from build123d import *

# Parameters (mm, degrees)
SKETCH1_W           = 5
SKETCH1_H           = 30
SKETCH1_W_2         = 30
SKETCH1_H_2         = 5.002209569
BOSS_EXTRUDE2_DEPTH = 5
FILLET1_R           = 5
FILLET2_R           = 2.5


with BuildPart() as part:
    # Sketch1 → Boss-Extrude2 (new body)
    with BuildSketch(Plane.XY):
        with BuildLine():
            Line((-77.831835846, -13.494171848), (-37.831835846, -13.494171848))
            ThreePointArc((-37.831835846, -13.494171848), (-30.760768034, -10.56523966), (-27.831835846, -3.494171848))
            Line((-27.831835846, -3.494171848), (-15.331835846, -3.494171848))
            Line((-15.331835846, -3.494171848), (-15.331835846, 36.505828152))
            Line((-15.331835846, 36.505828152), (-27.831835846, 36.505828152))
            ThreePointArc((-27.831835846, 36.505828152), (-30.760768034, 43.576895964), (-37.831835846, 46.505828152))
            Line((-37.831835846, 46.505828152), (-37.831835846, 59.005828152))
            Line((-37.831835846, 59.005828152), (-77.831835846, 59.005828152))
            Line((-77.831835846, 59.005828152), (-77.831835846, 46.505828152))
            ThreePointArc((-77.831835846, 46.505828152), (-84.902903658, 43.576895964), (-87.831835846, 36.505828152))
            Line((-87.831835846, 36.505828152), (-100.331835846, 36.505828152))
            Line((-100.331835846, 36.505828152), (-100.331835846, -3.494171848))
            Line((-100.331835846, -3.494171848), (-87.831835846, -3.494171848))
            ThreePointArc((-87.831835846, -3.494171848), (-84.902903658, -10.56523966), (-77.831835846, -13.494171848))
        make_face()
        with Locations((-90.331835846, 16.505828152)):
            Rectangle(SKETCH1_W, SKETCH1_H, mode=Mode.SUBTRACT)
        with Locations((-57.831835846, 49.006932937)):
            Rectangle(SKETCH1_W_2, SKETCH1_H_2, mode=Mode.SUBTRACT)
        with Locations((-25.331835846, 16.505828152)):
            Rectangle(SKETCH1_W, SKETCH1_H, mode=Mode.SUBTRACT)
    extrude(amount=BOSS_EXTRUDE2_DEPTH)

    # Fillet1
    fillet1_edges = [part.edges().sort_by_distance(p)[0] for p in [
        (-15.331835846, 36.505828152, 2.5),
        (-15.331835846, -3.494171848, 2.5),
        (-100.331835846, -3.494171848, 2.5),
        (-100.331835846, 36.505828152, 2.5),
        (-77.831835846, 59.005828152, 2.5),
        (-37.831835846, 59.005828152, 2.5),
    ]]
    fillet(fillet1_edges, radius=FILLET1_R)

    # Fillet2
    fillet2_edges = [part.edges().sort_by_distance(p)[0] for p in [
        (-22.831835846, 31.505828152, 2.5),
        (-22.831835846, 1.505828152, 2.5),
        (-92.831835846, 31.505828152, 2.5),
        (-92.831835846, 1.505828152, 2.5),
        (-72.831835846, 51.508037721, 2.5),
        (-42.831835846, 51.508037721, 2.5),
    ]]
    fillet(fillet2_edges, radius=FILLET2_R)


solid = part.part
Could you check a few things on this model? Use its own coordinates, in mm. A direction names the side the tool comes from. Give positions to 0.01 mm unless a question says otherwise; leave off trailing zeros. Order: outer loops, then holes, each group sorted by start corner. A loop starts at its lowest first (then second) coordinate and runs counter-clockwise, first axis right, second up. Notation, with made-up numbers: (15.5, 83) -> (74.5, 83) arc R17 cw to (74.5, 95) -> close; hole circle Ø8 at (77.25, 49). An arc over 180 degrees is marked (long way). Answer in a Markdown table with one row per item. Add a question column.
Item 1: Imagine slicing it at C-C (z = 2.25). Count the separate pieces of the cut face and the enclosed holes in it, and give its area (3 significant figures).
Item 2: For faces 1 (the flat face through (-77.832, 50, 2)), 2 (the flat face through (-24, -3.494, 2)), 3 (the flat face through (-58, 51.508, 2)), which set-ups out of +Z, -Z, +X, -X, +Y, -Y let a thin tool reach every point of the face, with its end or its side?
Item 3: Imagine slicing it at B-B (y = 20.5). List the corners of the cut face in (x, z) for me.
Item 4: I'm going to push flat-ended pins straight in: P1, Ø2.5, axis at x = -22.5, z = 1.5, coming from the +Y side; P2, Ø2.5, axis at x = -22.5, z = 3.5, coming from the -Y side; P3, Ø1.5, axis at x = -39, z = 4.5, coming from the +Y side. Where does each tip first touch, or does it pass through?
Item 5: Please list where these lines run through material, in increasing order: probe 1 along X at (y, z) = (4.5, 0.8); probe 2 along Y at (x, z) = (-66.5, 2.3); probe 3 along Y at (x, z) = (-95.5, 2).
Item 6: We'd pull the mould along X, two halves only. Please class faces 4 (the cylindrical face through (-76.41, 57.5, 2.54)), 5 (the flat face through (-72.832, 48, 2)), 6 (the flat face through (-58, 23, 0)), 7 (the cylindrical face through (-30.839, -10.643, 2.465)): pulls with the +X half, pulls with the -X half, needs draft (parallel to the pull), parting line crosses it, or undercut.
Item 7: Imagine slicing it at A-A (x = -58). List the corners of the cut face in (y, z) for me, and give its area (3 significant figures).
Item 8: Imagine slicing it at D-D (x = -44). List the corners of the cut face in (y, z) for me.
Result:
| question | item | result |
|---|---|---|
| 1 | separate pieces | 1 |
| 1 | enclosed holes | 3 |
| 1 | area | 4,540 mm2 |
| 2 | face 1 | +Z, -Z, -X, +Y |
| 2 | face 2 | +Z, -Z, +X, -Y |
| 2 | face 3 | +Z, -Z |
| 3 | outline | (-100.33, 0) -> (-92.83, 0) -> (-92.83, 5) -> (-100.33, 5) -> close; (-87.83, 0) -> (-27.83, 0) -> (-27.83, 5) -> (-87.83, 5) -> close; (-22.83, 0) -> (-15.33, 0) -> (-15.33, 5) -> (-22.83, 5) -> close |
| 4 | P1 | y = 36.51 |
| 4 | P2 | y = -3.49 |
| 4 | P3 | y = 57.94 |
| 5 | probe 1 | -100.33 to -92.83, -87.83 to -27.83, -22.83 to -15.33 |
| 5 | probe 2 | -13.49 to 46.51, 51.51 to 59.01 |
| 5 | probe 3 | -3.49 to 36.5 |
| 6 | face 4 | pulls with the -X half |
| 6 | face 5 | undercut |
| 6 | face 6 | needs draft |
| 6 | face 7 | pulls with the +X half |
| 7 | outline | (-13.49, 0) -> (46.51, 0) -> (46.51, 5) -> (-13.49, 5) -> close; (51.51, 0) -> (59.01, 0) -> (59.01, 5) -> (51.51, 5) -> close |
| 7 | area | 337 mm2 |
| 8 | outline | (-13.49, 0) -> (46.51, 0) -> (46.51, 5) -> (-13.49, 5) -> close; (51.12, 0) -> (59.01, 0) -> (59.01, 5) -> (51.12, 5) -> close |
